Study the drawing (mm; zero at the part's minimum x, y, z) and answer. A direction names the side the tool comes from. Give positions to 0.01 mm unless a question says otherwise; leave off trailing zeros. Loops run counter-clockwise (first coordinate to the right, second up) from the corner with the lowest first, then second, coordinate; pieces in that order, holes last. Notation, with made-up numbers: (86.5, 39.25) - (90.5, 39.25) arc R29 cw to (90.5, 60.25) - close; hole circle Ø3 at (25.25, 47). An arc over 180 degrees is marked (long way). Write item = value, one per line. Start each with the question number.
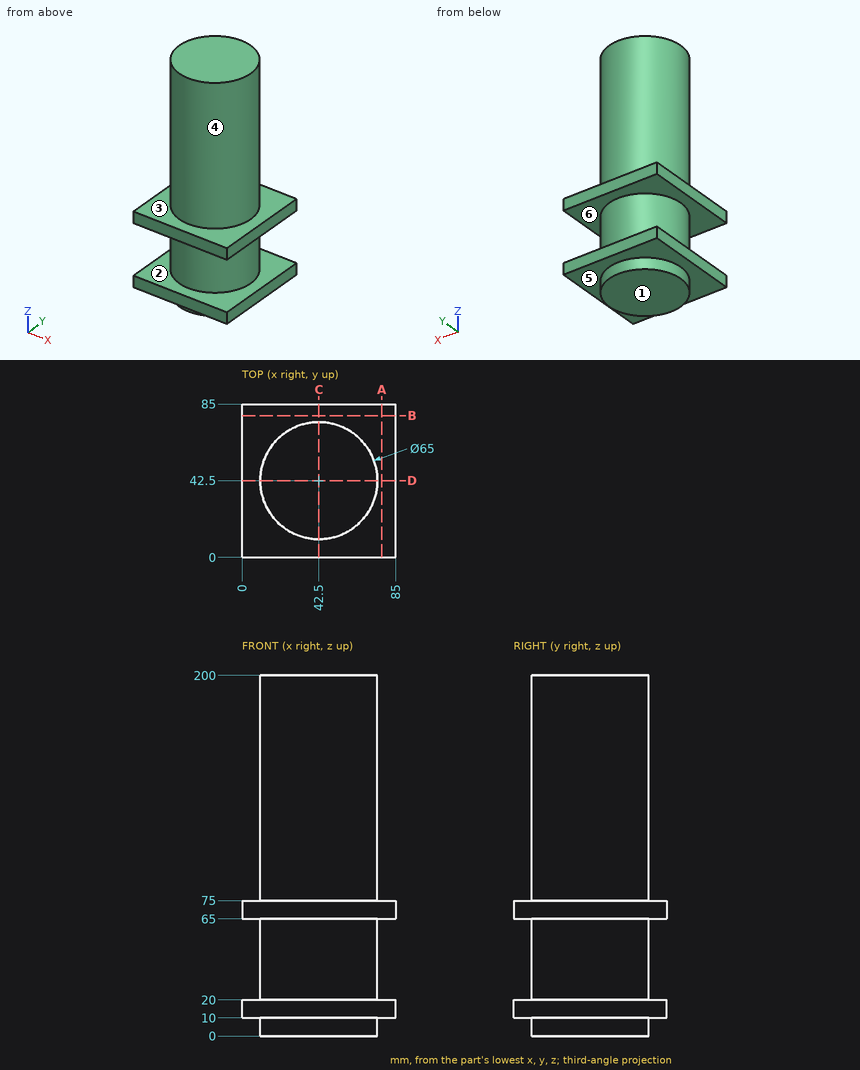
1. Consider line 1 along Z through (x, y) = (71.5, 79); line 2 along X through (y, z) = (40, 148.5); line 3 along X through (y, z) = (55.5, 123.5). Determine where each line is inside the solid, lowest interval first. Write a range as [from, to].
2. A tool of negligible diameter and unlimited length cuts with its end or side. For the marked faces 4, 5 and 6, from which of +Z, -Z, +X, -X, +Y, -Y can it reach the whole face along a straight path? Write none if from no direction.
3. Given P1, Ø8, axis at x = 46, z = 127, coming from the +Y side; P2, Ø2, axis at x = 55.5, z = 134, coming from the -Y side; P3, Ø8, axis at x = 67.5, z = 172.5, coming from the -Y side, each flat-ended and moving along its own axis, determine where each tip first touches the part or whether it passes through.
4. A cutting plane is placed at C-C on x = 42.5. Give the vertices of the cut face in (y, z), and give its area (3 significant figures).
5. A cutting plane is placed at A-A on x = 77.5. Give the vertices of the cut face in (y, z).
6. For a pull along Z with two mould halves and no side action, classify the marked faces 1, 2 and 3 as released by +Z, released by -Z, zero draft, split by the parting line, or undercut.
Reply:
q1.line_1 = [10, 20], [65, 75]
q1.line_2 = [10.1, 74.9]
q1.line_3 = [12.71, 72.29]
q2.face_4 = +Z
q2.face_5 = -Z
q2.face_6 = none
q3.P1 = 75
q3.P2 = 12.3
q3.P3 = 17.7
q4.outline = (0, 10) - (10, 10) - (10, 0) - (75, 0) - (75, 10) - (85, 10) - (85, 20) - (75, 20) - (75, 65) - (85, 65) - (85, 75) - (75, 75) - (75, 200) - (10, 200) - (10, 75) - (0, 75) - (0, 65) - (10, 65) - (10, 20) - (0, 20) - close
q4.area = 13,400 mm^2
q5.outline = (0, 10) - (85, 10) - (85, 20) - (0, 20) - close; (0, 65) - (85, 65) - (85, 75) - (0, 75) - close
q6.face_1 = released by -Z
q6.face_2 = undercut
q6.face_3 = released by +Z
